Print and shaded views of the part. All mm, measured from the part's lowest x, y and z. A direction names the side the tool comes from. Coordinates: 2 decimals unless noted, no trailing zeros. Loops run counter-clockwise (first coordinate to the right, second up) from the corner with the lowest first, then second, coordinate; pieces in that order, holes last.
1) Saw through at A-A, the plane y = 65. Write the cut outline in (x, z), and give its area (3 significant figures).
2) Saw through at B-B, the plane z = 65. Write the cut outline in (x, y), and give its area (4 significant figures).
3) Saw through at D-D, the plane z = 20.5. Write the cut outline in (x, y).
4) Saw through at C-C, the plane x = 227. Write the cut outline in (y, z).
5) Which spindle directions (+Z, -Z, +X, -X, +Y, -Y) get a long thin tool onto all of the face, cutting with end or side? Do the marked faces 1 and 2. Say none if no direction does.
6) Pin check, flat tips, straight feed: pin 1 Ø8 at (y, z) = (192, 99.5) entering from -X; pin 2 Ø5 at (y, z) = (193.5, 100) entering from +X; pin 3 Ø5 at (x, z) = (204, 42) entering from +Y. Stop position of each tip, or through.
7) Wall check: line 1 along Y through (x, z) = (218, 66); line 2 along Y through (x, z) = (81, 65); line 3 along Z through (x, y) = (150.5, 53). Give the ranges that are in metal, low to high.
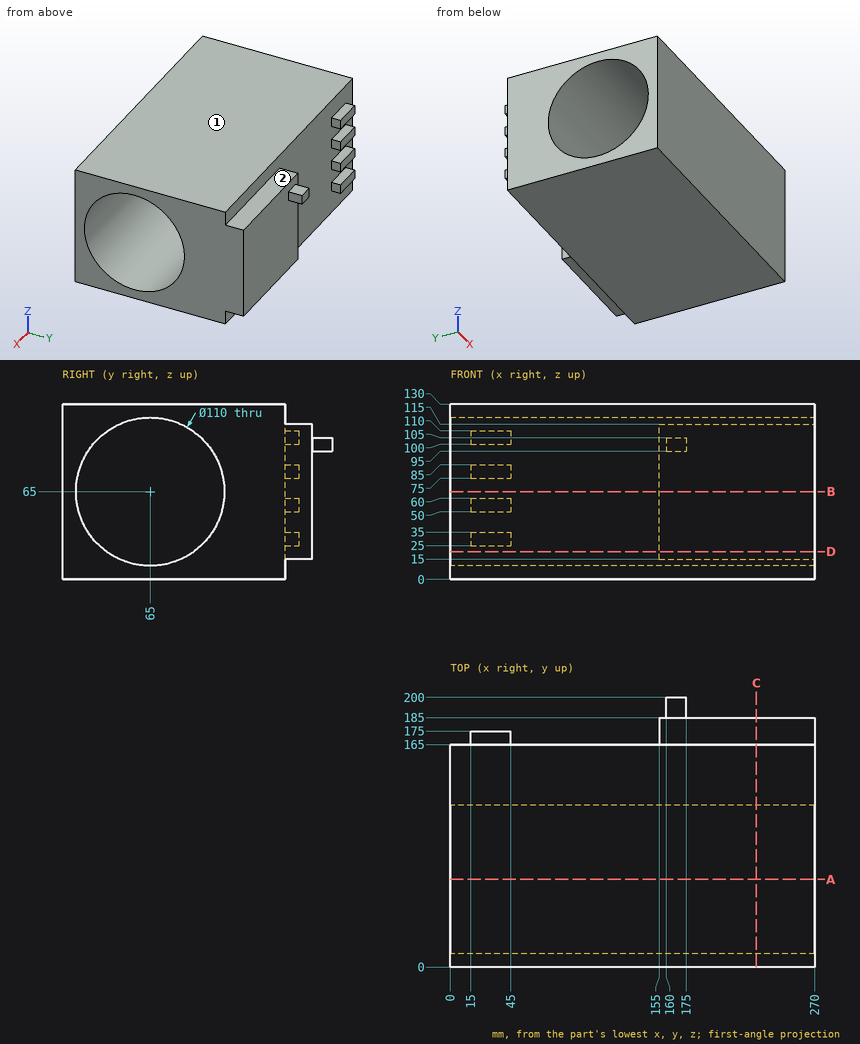
Data:
1. outline: (0, 0) - (270, 0) - (270, 10) - (0, 10) - close; (0, 120) - (270, 120) - (270, 130) - (0, 130) - close
1. area: 5,400 mm2
2. outline: (0, 0) - (270, 0) - (270, 10) - (0, 10) - close; (0, 120) - (270, 120) - (270, 185) - (155, 185) - (155, 165) - (0, 165) - close
2. area: 17,150 mm2
3. outline: (0, 0) - (270, 0) - (270, 32.68) - (0, 32.68) - close; (0, 97.32) - (270, 97.32) - (270, 185) - (155, 185) - (155, 165) - (0, 165) - close
4. outline: (0, 0) - (165, 0) - (165, 15) - (185, 15) - (185, 115) - (165, 115) - (165, 130) - (0, 130) - close; hole circle Ø110 at (65, 65)
5. face 1: +Z, +X, -X, +Y, -Y
5. face 2: +Z, +X, -X, +Y
6. pin 1: stops at x = 160
6. pin 2: stops at x = 175
6. pin 3: stops at y = 185
7. line 1: y = 0 to 10.01, 119.99 to 185
7. line 2: y = 0 to 10, 120 to 165
7. line 3: z = 0 to 11.33, 118.67 to 130
